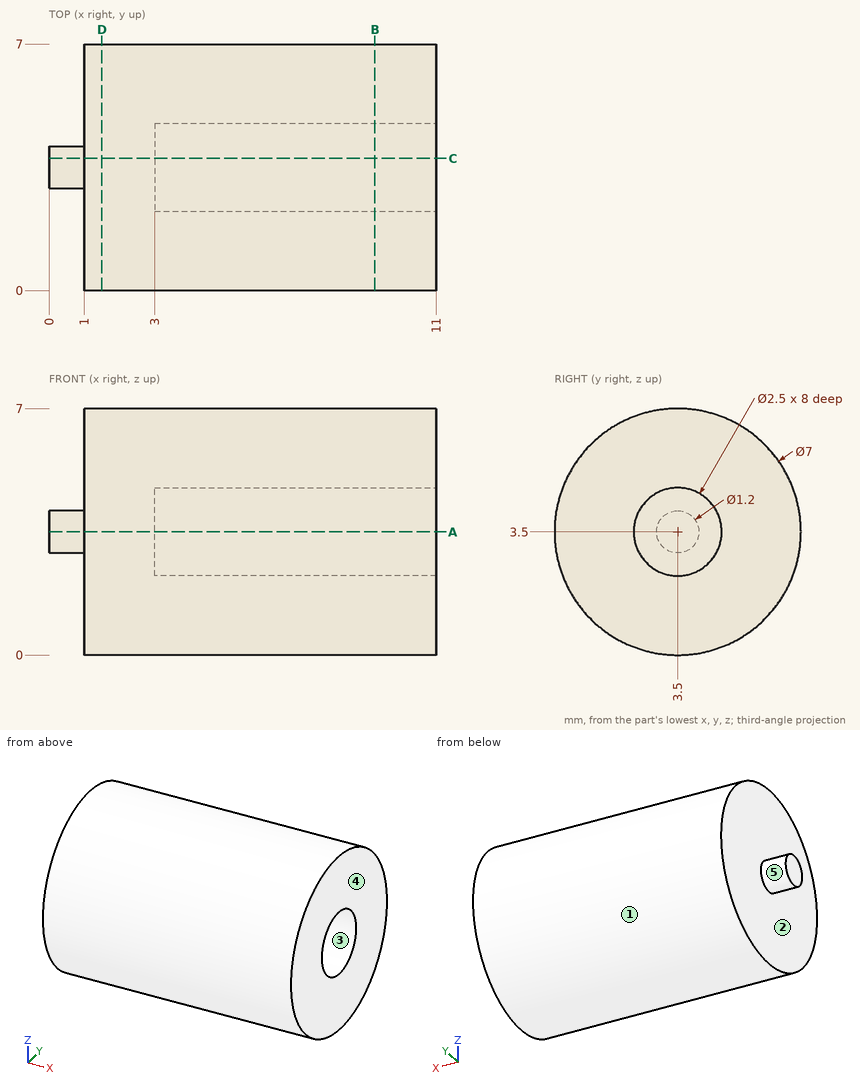
Geometry check sheet. Reference: drawing and pictorial views, mm from the part's lowest x, y, z. A direction names the side the tool comes from. Give positions to 0.01 mm unless a question says otherwise; leave off trailing zeros. Loops run counter-clockwise (first coordinate to the right, second up) from the corner with the lowest first, then second, coordinate; pieces in that order, holes last.
1. Section check C-C, the plane y = 3.75. Enter the section's corners in (x, z).
2. Section check B-B, the plane x = 9.25. Enter the section's corners in (y, z).
3. Section check A-A, the plane z = 3.5. Enter the section's corners in (x, y), then the cut area to 3 significant figures.
4. Set-up check for the marked faces 4 and 5: record each of +Z, -Z, +X, -X, +Y, -Y from which the full face is reachable in a straight line by a thin tool's end or side.
5. Go/stop test with flat-tipped pins: pin 1 Ø1.5 at (y, z) = (4.5, 5.5) entering from -X; pin 2 Ø0.8 at (y, z) = (3.5, 4) entering from +X; pin 3 Ø3 at (x, z) = (6.5, 1) entering from -Y. Record where each tip stops, or that it passes through.
6. Thickness scan on line 1 (X direction, y = 5.5, z = 1.75); line 2 (Z direction, x = 10.25, y = 2.75); line 3 (X direction, y = 4, z = 2.75). Record the ranges inside material, lowest first.
7. Mould release check, pull along Z, two halves, no side actions. Record for the marked faces 1, 2 and 3: released by +Z, released by -Z, zero draft, split by the parting line, or undercut.
8. Section check D-D, the plane x = 1.5. Enter the section's corners in (y, z), then the cut area to 3 significant figures.
Geometry says:
1. outline: (0, 2.95) - (1, 2.95) - (1, 0.01) - (11, 0.01) - (11, 2.28) - (3, 2.28) - (3, 4.72) - (11, 4.72) - (11, 6.99) - (1, 6.99) - (1, 4.05) - (0, 4.05) - close
2. outline: circle Ø7 at (3.5, 3.5); hole circle Ø2.5 at (3.5, 3.5)
3. outline: (0, 2.9) - (1, 2.9) - (1, 0) - (11, 0) - (11, 2.25) - (3, 2.25) - (3, 4.75) - (11, 4.75) - (11, 7) - (1, 7) - (1, 4.1) - (0, 4.1) - close
3. area: 51.2 mm2
4. face 4: +Z, -Z, +X, +Y, -Y
4. face 5: -X
5. pin 1: stops at x = 1
5. pin 2: stops at x = 3
5. pin 3: stops at y = 0.15
6. line 1: x = 1 to 11
6. line 2: z = 0.08 to 2.5, 4.5 to 6.92
6. line 3: x = 1 to 3
7. face 1: split by the parting line
7. face 2: zero draft
7. face 3: undercut
8. outline: circle Ø7 at (3.5, 3.5)
8. area: 38.5 mm2
